Study the drawing (mm; zero at the part's minimum x, y, z) and answer. A direction names the side the tool comes from. Give positions to 0.01 mm unless a question says otherwise; leave off trailing zeros. Write each loop counter-clockwise with the first axis right and the second up, starting at its lowest first coordinate (ties: lowest second). Pieces come first, ordered by that corner, then holes. Notation, with made-up numbers: (-29.75, 34) -> (4.25, 34) arc R15 cw to (4.25, 40) -> close; hole circle Ø4 at (-13, -17.75). An arc over 180 degrees is marked (long way). One line per question, with ' | ' between items.
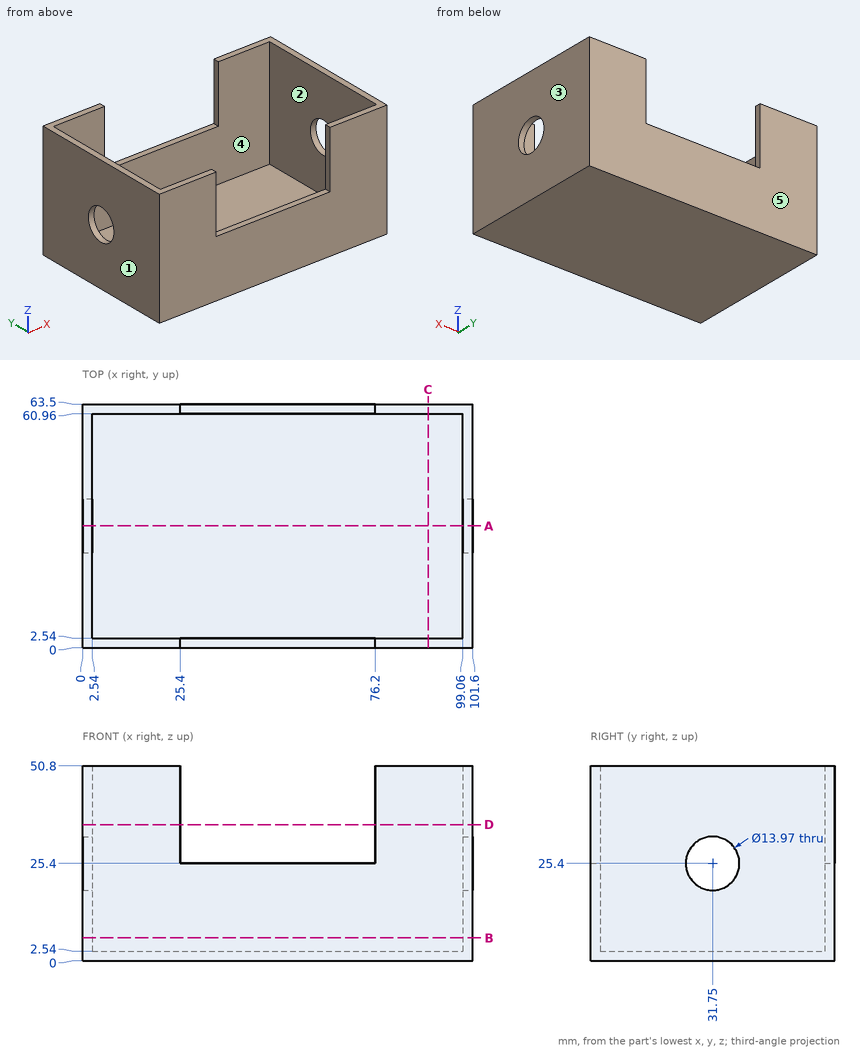
Item 1: Find section B-B (z = 6). Write down the section's boundary in (x, y), then the cut area to 3 significant figures.
Answers below:
outline: (0, 0) -> (101.6, 0) -> (101.6, 63.5) -> (0, 63.5) -> close; hole (2.54, 2.54) -> (99.06, 2.54) -> (99.06, 60.96) -> (2.54, 60.96) -> close | area: 813 mm²
Item 2: Find section A-A (y = 31.75). Write down the section's boundary in (x, z) (3 decimals).
Answers below:
outline: (0, 0) -> (101.6, 0) -> (101.6, 18.415) -> (99.06, 18.415) -> (99.06, 2.54) -> (2.54, 2.54) -> (2.54, 18.415) -> (0, 18.415) -> close; (0, 32.385) -> (2.54, 32.385) -> (2.54, 50.8) -> (0, 50.8) -> close; (99.06, 32.385) -> (101.6, 32.385) -> (101.6, 50.8) -> (99.06, 50.8) -> close
Item 3: Consider line 1 (X direction, y = 55.5, z = 8); line 2 (Z direction, x = 1.75, y = 31.75) (3 decimals); line 3 (Y direction, x = 90, z = 33). Determine where each line is inside the solid, lowest interval first. Write a range as [from, to].
Answers below:
line 1: [0, 2.54], [99.06, 101.6] | line 2: [0, 18.415], [32.385, 50.8] | line 3: [0, 2.54], [60.96, 63.5]
Item 4: Find section D-D (z = 35.5). Write down the section's boundary in (x, y), then the cut area to 3 significant figures.
Answers below:
outline: (0, 0) -> (25.4, 0) -> (25.4, 2.54) -> (2.54, 2.54) -> (2.54, 60.96) -> (25.4, 60.96) -> (25.4, 63.5) -> (0, 63.5) -> close; (76.2, 0) -> (101.6, 0) -> (101.6, 63.5) -> (76.2, 63.5) -> (76.2, 60.96) -> (99.06, 60.96) -> (99.06, 2.54) -> (76.2, 2.54) -> close | area: 555 mm²
Item 5: A tool of negligible diameter and unlimited length cuts with its end or side. For the marked faces 1 and 2, from which of +Z, -Z, +X, -X, +Y, -Y can it reach the whole face along a straight path? Write none if from no direction.
Answers below:
face 1: +Z, -Z, -X, +Y, -Y | face 2: +Z
Item 6: Determine the mould class of the marked faces 3, 4 and 5 for opening direction X: pulls with the +X half, pulls with the -X half, needs draft (parallel to the pull), parting line crosses it, or undercut.
Answers below:
face 3: pulls with the +X half | face 4: undercut | face 5: needs draft
Item 7: Flat-ended cylindrical pins translate along their axes: pin 1 (2 mm diameter, centred on x = 50, y = 0.5, fed in from +Z); pin 2 (1.5 mm diameter, centred on x = 63.5, y = 45, fed in from +Z); pin 3 (11 mm diameter, centred on y = 31.75, z = 25.4, fed in from -X). Find the tip coordinate at first contact, or state that the pin passes through.
Answers below:
pin 1: z = 25.4 | pin 2: z = 2.54 | pin 3: through
Item 8: Find section C-C (x = 90). Write down the section's boundary in (y, z), then the cut area to 3 significant figures.
Answers below:
outline: (0, 0) -> (63.5, 0) -> (63.5, 50.8) -> (60.96, 50.8) -> (60.96, 2.54) -> (2.54, 2.54) -> (2.54, 50.8) -> (0, 50.8) -> close | area: 406 mm²
